Verification items for this drawing (mm, ordinates from the low corner). Round coordinates to 2 decimals unless told otherwise and drop trailing zeros. Loops run counter-clockwise (first coordinate to the right, second up) from the corner with the lowest first, then second, coordinate; pieces in that order, holes last. Notation, with made-up numbers: (82, 31) - (87, 31) arc R7 cw to (87, 43) - close; hole circle Ø7 at (41, 68.5). An arc over 180 degrees is marked (long way). Put each result on its own line as item: value.
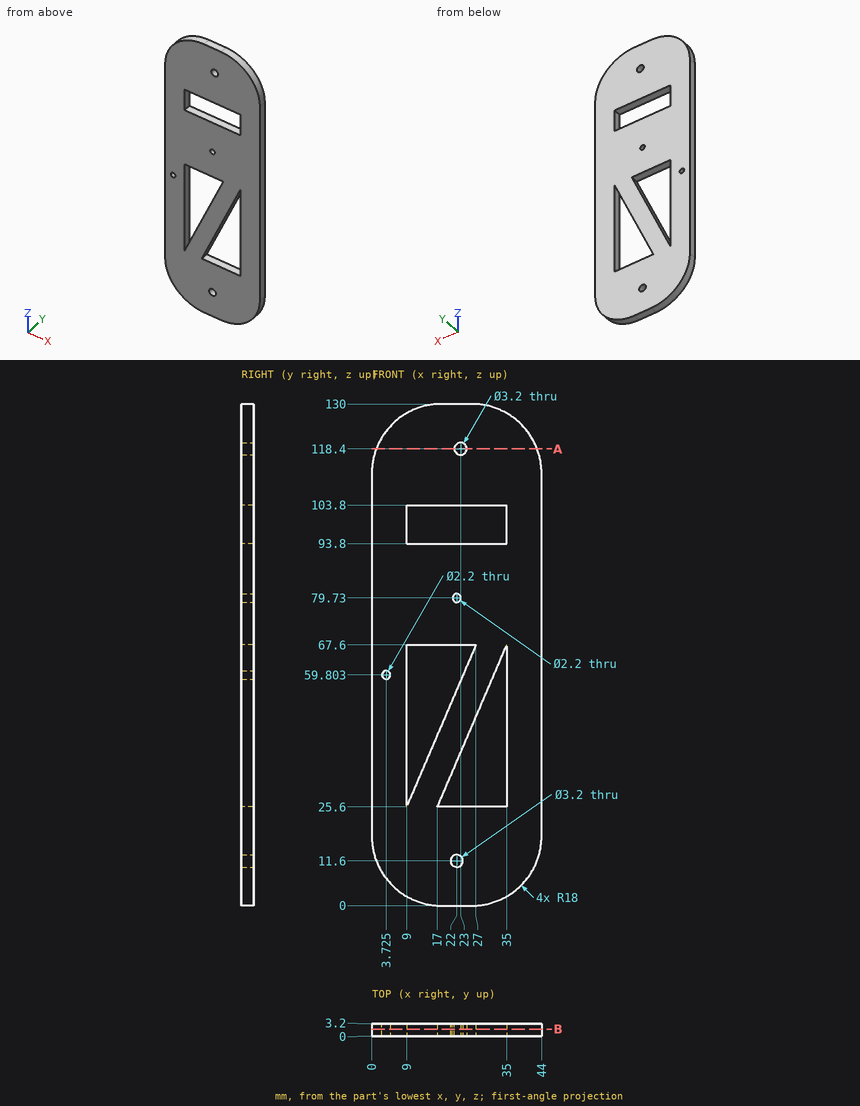
Item 1: Section check A-A on z = 118.4. Enter the section's corners in (x, y), then the cut area to 3 significant figures.
Filled sheet:
outline: (1.18, 0) - (21.4, 0) - (21.4, 3.2) - (1.18, 3.2) - close; (24.6, 0) - (42.82, 0) - (42.82, 3.2) - (24.6, 3.2) - close
area: 123 mm²
Item 2: Thickness scan on line 1 (Z direction, x = 19, y = 1) (1 decimal); line 2 (Z direction, x = 13, y = 1.9) (1 decimal); line 3 (X direction, y = 1.55, z = 31) (1 decimal). Record the ranges inside material, lowest first. Write a range as from..to.
Filled sheet:
line 1: 0..25.6, 30.3..48.9, 67.6..93.8, 103.8..130
line 2: 0.7..34.9, 67.6..93.8, 103.8..129.3
line 3: 0..9, 11.3..19.3, 35..44
Item 3: Section check B-B on y = 1.75. Enter the section's corners in (x, z) (1 decimal).
Filled sheet:
outline: (0, 18) arc R18 ccw to (18, 0) - (26, 0) arc R18 ccw to (44, 18) - (44, 112) arc R18 ccw to (26, 130) - (18, 130) arc R18 ccw to (0, 112) - close; hole circle Ø2.2 at (3.7, 59.8); hole (9, 25.6) - (27, 67.6) - (9, 67.6) - close; hole (9, 93.8) - (35, 93.8) - (35, 103.8) - (9, 103.8) - close; hole (17, 25.6) - (35, 25.6) - (35, 67.6) - close; hole circle Ø3.2 at (22, 11.6); hole circle Ø2.2 at (22, 79.7); hole circle Ø3.2 at (23, 118.4)
Item 4: Go/stop test with a flat-tipped pin: pin 1 (3 mm diameter, centred on x = 23, z = 118.4, fed in from +Y). Record where the tip stops, or that it passes through.
Filled sheet:
pin 1: through
